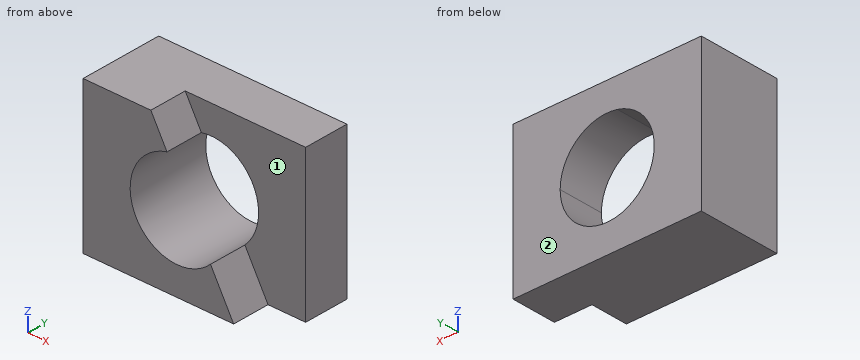
from build123d import *

# Parameters (mm, degrees)
F0_W     = 100
F0_H     = 80
F1_DEPTH = 22
F3_DEPTH = 20
F5_DEPTH = 44.001


with BuildPart() as f1:
    # F0 (on Front) → F1 (new body, symmetric)
    with BuildSketch(Plane.XZ):
        Rectangle(F0_W, F0_H)
    extrude(amount=F1_DEPTH, both=True)

    # F2 (on face) → F3 (cut)
    with BuildSketch(Plane.XZ.offset(22)):
        Polygon((-14, 40), (30, -40), (50, -40), (50, 40), align=None)
    extrude(amount=-F3_DEPTH, mode=Mode.SUBTRACT)

    # F4 (on face) → F5 (cut, through all)
    with BuildSketch(Plane.XZ.offset(22)):
        with BuildLine():
            ThreePointArc((17.706716, -17.648575), (23.104847, -9.548091), (25, 0))
            ThreePointArc((25, 0), (15.64343, 19.500848), (-5.422647, 24.404813))
            Line((-5.422647, 24.404813), (17.706716, -17.648575))
        make_face()
        with BuildLine():
            Line((17.706716, -17.648575), (-5.422647, 24.404813))
            ThreePointArc((-5.422647, 24.404813), (-21.905398, -12.047969), (17.706716, -17.648575))
        make_face()
    extrude(amount=-F5_DEPTH, mode=Mode.SUBTRACT)


solid = f1.part
Design review of the part built by this model. Coordinates are the model's own, in mm. Face numbers are marked on the shaded views. A direction names the side the tool comes from. Round coordinates to 2 decimals unless told otherwise and drop trailing zeros. Write each loop counter-clockwise with the first axis right and the second up, starting at its lowest first coordinate (ties: lowest second). Pieces come first, ordered by that corner, then holes. Notation, with made-up numbers: (86, 84) -> (112, 84) arc R30 ccw to (112, 111) -> close; hole circle Ø6 at (60, 37). An arc over 180 degrees is marked (long way). One line per question, with ' | ' between items.
(1) Take a section at C-C, the plane z = -21. State the section outline as (x, y) points, and give its area (3 significant figures).
Result sheet:
outline: (-50, -22) -> (-13.56, -22) -> (-13.56, 22) -> (-50, 22) -> close; (13.56, -22) -> (19.55, -22) -> (19.55, -2) -> (50, -2) -> (50, 22) -> (13.56, 22) -> close | area: 2,600 mm2
(2) Insertion check: P1, Ø2, axis at y = -13.5, z = 21.5, coming from the +X side. The pin has a flat end and moves straight along its axis. Give the tip position at first contact, or say it passes through.
Result sheet:
P1: x = -10.9
(3) Take a section at A-A, the plane x = 0. State the section outline as (y, z) points.
Result sheet:
outline: (-22, -40) -> (22, -40) -> (22, -25) -> (-22, -25) -> close; (-2, 25) -> (22, 25) -> (22, 40) -> (-2, 40) -> close
(4) Take a section at B-B, the plane y = 4. State the section outline as (x, z) points.
Result sheet:
outline: (-50, -40) -> (50, -40) -> (50, 40) -> (-50, 40) -> close; hole (17.71, -17.65) arc R25 ccw to (25, 0) arc R25 ccw (long way) to start
(5) Wall thickness on line 1 (Z direction, x = 0, y = 10); line 2 (X direction, y = 15, z = 0.5) (3 decimals); line 3 (Y direction, x = 32, z = 18.5): over which ranges is each line inside the solid? List them lowest first. Write a range as [from, to].
Result sheet:
line 1: [-40, -25], [25, 40] | line 2: [-50, -24.995], [24.995, 50] | line 3: [-2, 22]
(6) Machinability: for the marked faces 1 and 2, which of the approach directions +Z, -Z, +X, -X, +Y, -Y give a long, thin tool a straight path to every point of the face, cutting with its end or side? Answer none if there is none.
Result sheet:
face 1: +Z, +X, -Y | face 2: +Z, -Z, +X, -X, +Y
(7) Take a section at D-D, the plane x = 32.5. State the section outline as (y, z) points.
Result sheet:
outline: (-2, -40) -> (22, -40) -> (22, 40) -> (-2, 40) -> close
